CAD build for the part. Positions are in the model's coordinates, mm. Face numbers are marked on the shaded views. Round coordinates to 2 decimals unless told otherwise and drop trailing zeros. Order: outer loops, then holes, each group sorted by start corner. A loop starts at its lowest first (then second) coordinate and runs counter-clockwise, first axis right, second up. Notation, with made-up numbers: M 80,56.5 L 85,56.5 A27 cw 85,80.5 Z; hole C -35,-1 d4. An arc over 180 degrees is marked long. Answer as CSV lines item,"result". Start each with the question number.
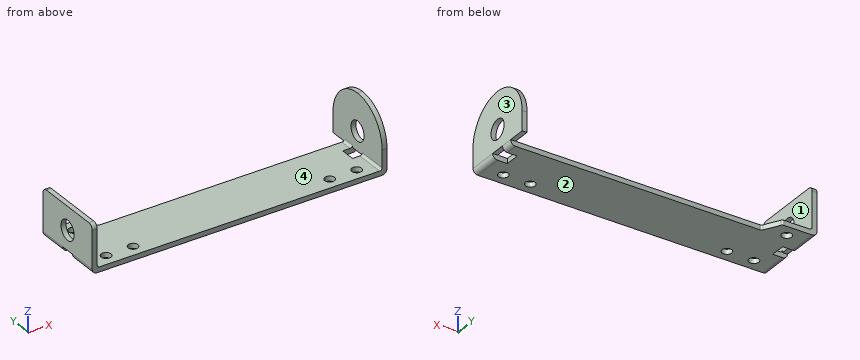
```python
from build123d import *

# Parameters (mm, degrees)
F0_W      = 60
F0_H      = 15
F1_DEPTH  = 1
F2_W      = 1
F2_H      = 15
F3_DEPTH  = 8.7
F4_W      = 1
F4_H      = 15
F5_DEPTH  = 11.5
F6_W      = 3
F6_H      = 3
F6_R      = 1
F7_DEPTH  = 1
F8_R      = 7.49999
F9_R      = 0.5
F10_R     = 1
F11_R     = 2
F12_DEPTH = 60.001


# Not quite as in the source:
# - a fillet or chamfer is up to 0.001 mm smaller than in the source, because OpenCascade refuses the exact size


with BuildPart() as f1:
    # F0 (on Top) → F1 (new body)
    with BuildSketch(Plane.XY):
        with Locations((30, 7.5)):
            Rectangle(F0_W, F0_H)
    extrude(amount=F1_DEPTH)

    # F2 (on face) → F3 (join)
    with BuildSketch(Plane.XY.offset(1)):
        with Locations((0.5, 7.5)):
            Rectangle(F2_W, F2_H)
    extrude(amount=F3_DEPTH)

    # F4 (on face) → F5 (join)
    with BuildSketch(Plane.XY.offset(1)):
        with Locations((59.5, 7.5)):
            Rectangle(F4_W, F4_H)
    extrude(amount=F5_DEPTH)

    # F6 (on face) → F7 (cut, through all)
    with BuildSketch(Plane(origin=(0, 0, 0), x_dir=(1, 0, 0), z_dir=(0, 0, -1))):
        with Locations((1.5, -7.5)):
            Rectangle(F6_W, F6_H)
        with Locations((4.5, -2.5)):
            Circle(F6_R)
        with Locations((10, -2.5)):
            Circle(F6_R)
        with Locations((50, -2.5)):
            Circle(F6_R)
        with Locations((55.5, -2.5)):
            Circle(F6_R)
        with Locations((58.5, -7.5)):
            Rectangle(F6_W, F6_H)
        with Locations((4.5, -12.5)):
            Circle(F6_R)
        Polygon((9, -11.5), (7, -15), (60, -15), (60, -11.5), align=None)
    extrude(amount=-F7_DEPTH, mode=Mode.SUBTRACT)

    # F8 (radius 7.5 in the source; OpenCascade refuses exactly that, so slightly less here)
    f8_edges = [f1.edges().sort_by_distance(p)[0] for p in [
        (59.5, 0, 12.5),
        (59.5, 15, 12.5),
    ]]
    fillet(f8_edges, radius=F8_R)

    # F9
    f9_edges = [f1.edges().sort_by_distance(p)[0] for p in [
        (59, 3, 1),
        (59, 10.25, 1),
        (1, 3, 1),
        (1, 12, 1),
        (7, 15, 0.5),
        (9, 11.5, 0.5),
    ]]
    fillet(f9_edges, radius=F9_R)

    # F10
    f10_edges = [f1.edges().sort_by_distance(p)[0] for p in [
        (60, 10.25, 0),
        (60, 3, 0),
        (0, 12, 0),
        (0, 3, 0),
        (0.5, 0, 9.7),
        (0.5, 15, 9.7),
    ]]
    fillet(f10_edges, radius=F10_R)

    # F11 (on face) → F12 (cut, through all)
    with BuildSketch(Plane.YZ.offset(60)):
        with Locations((7.5, 5)):
            Circle(F11_R)
    extrude(amount=-F12_DEPTH, mode=Mode.SUBTRACT)


solid = f1.part
```
Q1. Band-saw the part on C-C, the plane z = 8. Write the cut outline in (x, y), then the cut area to 3 significant figures.
Q2. Band-saw the part on D-D, the plane y = 12.5. Write the cut outline in (x, z).
Q3. Band-saw the part on B-B, the plane y = 2.5. Write the cut outline in (x, z).
Q4. Mould opens along X. For the marked faces 1, 2, 3 and 4 say: +X half, -X half, draft (parallel to the pull), parting line (faces both ways), or undercut.
Q5. Band-saw the part on A-A, the plane x = 4.5. Write the cut outline in (y, z).
Q6. Drop flat-ended pins along their axis: P1, Ø1.1, axis at x = 0.5, y = 8, coming from the +Z side; P2, Ø0.8, axis at x = 0.5, y = 8, coming from the -Z side; P3, Ø3, axis at x = 4.5, y = 2.5, coming from the +Z side. Give the stop position or say it passes through.
Q7. Probe line 1 along Y through (x, z) = (4.5, 0.6); line 2 along Y through (x, z) = (10, 0.35); line 3 along X through (y, z) = (12.5, 4.25). List the from-to ranges inside material, lowest first. Write a range as from..to.
Answer:
1,outline,"M 0,0 L 1,0 L 1,15 L 0,15 Z; M 59,0.63 L 60,0.63 L 60,14.37 L 59,14.37 Z"
1,area,"28.7 mm^2"
2,outline,"M 0,1 A1 ccw 1,0 L 3.5,0 L 3.5,1 L 1.5,1 A0.5 cw 1,1.5 L 1,9.7 L 0,9.7 Z; M 5.5,0 L 8.43,0 L 8.43,1 L 5.5,1 Z; M 59,1 L 60,1 L 60,10.59 L 59,10.59 Z"
3,outline,"M 0,1 A1 ccw 1,0 L 3.5,0 L 3.5,1 L 1.5,1 A0.5 cw 1,1.5 L 1,9.7 L 0,9.7 Z; M 5.5,0 L 9,0 L 9,1 L 5.5,1 Z; M 11,0 L 49,0 L 49,1 L 11,1 Z; M 51,0 L 54.5,0 L 54.5,1 L 51,1 Z; M 56.5,0 L 59,0 A1 ccw 60,1 L 60,10.59 L 59,10.59 L 59,1.5 A0.5 cw 58.5,1 L 56.5,1 Z"
4,face 1,"undercut"
4,face 2,"draft"
4,face 3,"+X half"
4,face 4,"undercut"
5,outline,"M 0,0 L 1.5,0 L 1.5,1 L 0,1 Z; M 3.5,0 L 11.5,0 L 11.5,1 L 3.5,1 Z; M 13.5,0 L 15,0 L 15,1 L 13.5,1 Z"
6,P1,"stops at z = 9.7"
6,P2,"stops at z = 1"
6,P3,"stops at z = 1"
7,line 1,"y = 0..1.5, 3.5..11.5, 13.5..15"
7,line 2,"y = 0..1.5, 3.5..11.5"
7,line 3,"x = 0..1, 59..60"
